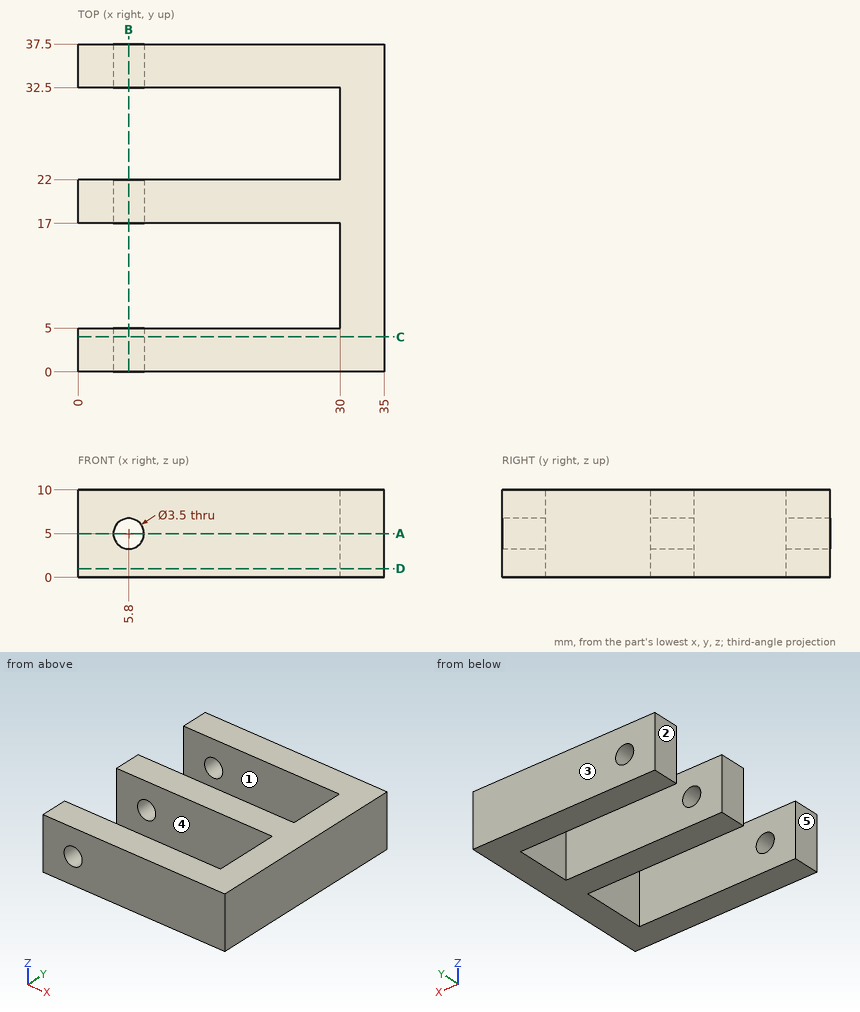
Could you check a few things on this drawing? It's one solid part, dimensions in mm from its lowest x, y, z. A direction names the side the tool comes from. Round coordinates to 2 decimals unless told otherwise and drop trailing zeros. Write each loop counter-clockwise with the first axis right and the second up, starting at its lowest first coordinate (ties: lowest second). Pieces come first, ordered by that corner, then holes. Notation, with made-up numbers: (-1.75, -27.5) -> (38.25, -27.5) arc R15 ccw to (38.25, -19.5) -> close; hole circle Ø1 at (31, -3). An arc over 180 degrees is marked (long way). Use one line per item in the form item = value. Start each with the question number.
Q1. Imagine slicing it at A-A (z = 5). Please give me the cut outline in (x, y).
Q2. Imagine slicing it at D-D (z = 1). Please give me the cut outline in (x, y), then the cut area to 4 significant figures.
Q3. I'm going to push flat-ended pins straight in: P1, Ø5, axis at y = 14, z = 7, coming from the -X side; P2, Ø5, axis at x = 19, y = 8.5, coming from the -Z side. Where does each tip first touch, or does it pass through?
Q4. Imagine slicing it at B-B (x = 5.8). Please give me the cut outline in (y, z), then the cut area to 3 significant figures.
Q5. Imagine slicing it at C-C (y = 4). Please give me the cut outline in (x, z).
Q6. We'd pull the mould along Y, two halves only. Please class the marked faces 1, 2 and 3: +Y half, -Y half, draft (parallel to the pull), parting line (faces both ways), or undercut.
Q7. If I drill on probe 1 along Y at (x, z) = (24.5, 3); probe 2 along X at (y, z) = (3.6, 5); probe 3 along X at (y, z) = (7.5, 5.75), over which ranges is the centre line in solid material (lowest first)? Write a range as [from, to].
Q8. Which directions (+Z, -Z, +X, -X, +Y, -Y) give clear straight access to the entire face, cutting with the end or side of a thin tool? Please do the marked faces 4 and 5.
Worked out:
q1.outline = (0, 0) -> (4.05, 0) -> (4.05, 5) -> (0, 5) -> close; (0, 17) -> (4.05, 17) -> (4.05, 22) -> (0, 22) -> close; (0, 32.5) -> (4.05, 32.5) -> (4.05, 37.5) -> (0, 37.5) -> close; (7.55, 0) -> (35, 0) -> (35, 37.5) -> (7.55, 37.5) -> (7.55, 32.5) -> (30, 32.5) -> (30, 22) -> (7.55, 22) -> (7.55, 17) -> (30, 17) -> (30, 5) -> (7.55, 5) -> close
q2.outline = (0, 0) -> (35, 0) -> (35, 37.5) -> (0, 37.5) -> (0, 32.5) -> (30, 32.5) -> (30, 22) -> (0, 22) -> (0, 17) -> (30, 17) -> (30, 5) -> (0, 5) -> close
q2.area = 637.5 mm^2
q3.P1 = 30
q3.P2 = through
q4.outline = (0, 0) -> (5, 0) -> (5, 3.25) -> (0, 3.25) -> close; (0, 6.75) -> (5, 6.75) -> (5, 10) -> (0, 10) -> close; (17, 0) -> (22, 0) -> (22, 3.25) -> (17, 3.25) -> close; (17, 6.75) -> (22, 6.75) -> (22, 10) -> (17, 10) -> close; (32.5, 0) -> (37.5, 0) -> (37.5, 3.25) -> (32.5, 3.25) -> close; (32.5, 6.75) -> (37.5, 6.75) -> (37.5, 10) -> (32.5, 10) -> close
q4.area = 97.5 mm^2
q5.outline = (0, 0) -> (35, 0) -> (35, 10) -> (0, 10) -> close; hole circle Ø3.5 at (5.8, 5)
q6.face_1 = undercut
q6.face_2 = draft
q6.face_3 = +Y half
q7.probe_1 = [0, 5], [17, 22], [32.5, 37.5]
q7.probe_2 = [0, 4.05], [7.55, 35]
q7.probe_3 = [30, 35]
q8.face_4 = +Z, -Z, -X
q8.face_5 = +Z, -Z, -X, +Y, -Y
